Check sheet for the modelled part. Datum: model origin and axes. Units: mm. Coordinates: 2 decimals unless noted, no trailing zeros. Write each loop counter-clockwise with the first axis right and the second up, starting at its lowest first coordinate (ties: lowest second). Pieces come first, ordered by that corner, then holes. Notation, with made-up numbers: M 83.25,17.5 L 130.25,17.5 A15 ccw 130.25,37.5 Z; hole C 81.5,55.25 d4. An arc over 180 degrees is marked long. Answer as CSV lines item,"result".
from build123d import *

# Parameters (mm, degrees)
F3_DEPTH = 25
F4_COUNT = 25


with BuildPart() as f1:
    # F0 (on Front) → F1 (revolve)
    with BuildSketch(Plane.XZ):
        with BuildLine():
            Line((5, 15.7740319341), (5, 21.2740319341))
            ThreePointArc((5, 21.2740319341), (4.8535533906, 21.6275853247), (4.5, 21.7740319341))
            Line((4.5, 21.7740319341), (3.1358124877, 21.7740319341))
            ThreePointArc((3.1358124877, 21.7740319341), (2.7822590971, 21.6275853247), (2.6358124877, 21.2740319341))
            Line((2.6358124877, 21.2740319341), (2.6358124877, 20.2740319341))
            Line((2.6358124877, 20.2740319341), (-2.3641875123, 20.2740319341))
            Line((-2.3641875123, 20.2740319341), (-2.3641875123, 21.2740319341))
            ThreePointArc((-2.3641875123, 21.2740319341), (-2.5106341217, 21.6275853247), (-2.8641875123, 21.7740319341))
            Line((-2.8641875123, 21.7740319341), (-4.5107149994, 21.7740319341))
            ThreePointArc((-4.5107149994, 21.7740319341), (-4.8604185225, 21.6313937199), (-5.0105977014, 21.2848617178))
            Line((-5.0105977014, 21.2848617178), (-5.1299878986, 15.7740319341))
            Line((-5.1299878986, 15.7740319341), (0, 15.7740319341))
            Line((0, 15.7740319341), (5, 15.7740319341))
        make_face()
    revolve(axis=Axis((-3.1572775915, 0, 4.2740319341), (-1, 0, 0)))

    # F2 (on face) → F3 (cut)
    with BuildSketch(Plane.YZ.offset(5)):
        with BuildLine():
            Line((0.5, 16.7740319341), (0, 16.7740319341))
            Line((0, 16.7740319341), (-0.5, 16.7740319341))
            Line((-0.5, 16.7740319341), (-0.8761352278, 15.740608889))
            ThreePointArc((-0.8761352278, 15.740608889), (0, 15.7740319341), (0.8761352278, 15.740608889))
            Line((0.8761352278, 15.740608889), (0.5, 16.7740319341))
        make_face()
    f3 = extrude(amount=-F3_DEPTH, mode=Mode.SUBTRACT)

    # F4: F3 ×25 about axis
    f4_axis = Axis((-5.1299878986, 0, 4.2740319341), (1, 0, 0))
    for i in range(1, F4_COUNT):
        add(f3.rotate(f4_axis, i * 360 / F4_COUNT), mode=Mode.SUBTRACT)


solid = f1.part
1) Mould release check, pull along Z, two halves, no side actions. Record for faces 1 (the face through (3.81, -10.65, -9.61)), 2 (the face through (0.01, 10.94, 0.73)): pulls with the +Z half, pulls with the -Z half, needs draft (parallel to the pull), parting line crosses it, or undercut.
Answer key:
face 1,"parting line crosses it"
face 2,"undercut"
2) Section check A-A, the plane y = 0. Record the boundary of the cut face in (x, z), plus the area to 3 significant figures.
Answer key:
outline,"M -5.13,-7.23 L -5.01,-12.74 A0.5 ccw -4.51,-13.23 L -2.86,-13.23 A0.5 ccw -2.36,-12.73 L -2.36,-11.73 L 2.64,-11.73 L 2.64,-12.73 A0.5 ccw 3.14,-13.23 L 4.5,-13.23 A0.5 ccw 5,-12.73 L 5,-7.23 Z; M -5.11,16.77 L 5,16.77 L 5,21.27 A0.5 ccw 4.5,21.77 L 3.14,21.77 A0.5 ccw 2.64,21.27 L 2.64,20.27 L -2.36,20.27 L -2.36,21.27 A0.5 ccw -2.86,21.77 L -4.51,21.77 A0.5 ccw -5.01,21.28 Z"
area,"95.2 mm2"
3) Depth check by flat-ended pin: P1, Ø3, axis at x = -2, z = -4, coming from the -Y side; P2, Ø3, axis at x = 0.5, y = -6, coming from the -Z side; P3, Ø1.5, axis at x = 0.5, y = -1, coming from the -Z side. Enter the tip coordinate at first touch or a pass-through.
Answer key:
P1,"stops at y = -16.04"
P2,"stops at z = -11.08"
P3,"stops at z = -11.72"
4) Thickness scan on line 1 along Y through (x, z) = (4.25, 4); line 2 along Z through (x, y) = (4.25, 10.5); line 3 along Z through (x, y) = (-2.5, 9.5). Record the ranges inside material, lowest first.
Answer key:
line 1,"y = -17.5 to -11.5, 11.5 to 17.5"
line 2,"z = -9.73 to -1.45, 8.96 to 10.13, 11.06 to 18.27"
line 3,"z = -10.24 to -3.85, -2.54 to -2.21, 11.22 to 18.78"
